Here's how the part is built. I have some questions about the finished solid (model axes, mm). A direction names the side the tool comes from. Round coordinates to 2 decimals unless told otherwise and drop trailing zeros. Loops run counter-clockwise (first coordinate to the right, second up) from the corner with the lowest first, then second, coordinate; pieces in that order, holes last. Notation, with made-up numbers: (56, 52) -> (72, 52) arc R30 cw to (72, 80) -> close; hole circle Ø5 at (69.5, 31.25). An arc over 180 degrees is marked (long way). Use one line per item in the form item = value. Start each with the question number.
Item 1: If we section it at C-C (z = 12.5): Write out the boundary of the cut face in (x, y), then the cut area to 3 significant figures.
Item 2: If we section it at D-D (z = 5): Write out the boundary of the cut face in (x, y), then the cut area to 3 significant figures.
Item 3: I'm going to push flat-ended pins straight in: pin 1 Ø1.5 at (y, z) = (-2.5, 12.5) entering from +X; pin 2 Ø8 at (y, z) = (-4.5, 9.5) entering from -X; pin 3 Ø3 at (x, z) = (2, 3.5) entering from +Y. Where does each tip first touch, or does it pass through?
Item 4: For faces 4 (the face through (-2.8, 0.1, 17.1)), 5 (the face through (-2.539, 1.947, 1.972)), which set-ups out of +Z, -Z, +X, -X, +Y, -Y let a thin tool reach every point of the face, with its end or its side?
Item 5: If I drill on L1, parallel to Y at x = 0, z = 13.75; L2, parallel to Y at x = 0, z = 8; L3, parallel to X at y = 1, z = 5.25, over which ranges is the centre line in solid material (lowest first)? Write a range as [from, to].
Item 6: Thinking about a two-plate mould opening in Y: for faces 1 (the face through (6.466, -2.681, 11.339)), 2 (the face through (1.5, -3, 0)), 3 (the face through (-3, 0, 7)), which applies, released by +Y, released by -Y, zero draft, split by the parting line, or undercut?
Item 7: If we section it at A-A (x = 0): Write out the boundary of the cut face in (y, z).
```python
from build123d import *

# Parameters (mm, degrees)
F0_R     = 7
F1_DEPTH = 23
F2_R     = 2.8
F3_DEPTH = 23.001
F4_R     = 3.2
F5_DEPTH = 4
F6_R     = 3
F7_DEPTH = 7


with BuildPart() as f1:
    # F0 (on Top) → F1 (new body)
    with BuildSketch(Plane.XY):
        Circle(F0_R)
    extrude(amount=F1_DEPTH)

    # F2 (on face) → F3 (cut, through all)
    with BuildSketch(Plane.XY.offset(23)):
        Circle(F2_R)
    extrude(amount=-F3_DEPTH, mode=Mode.SUBTRACT)

    # F4 (on face) → F5 (cut)
    with BuildSketch(Plane(origin=(0, 0, 0), x_dir=(1, 0, 0), z_dir=(0, 0, -1))):
        Circle(F4_R)
    extrude(amount=-F5_DEPTH, mode=Mode.SUBTRACT)

    # F6 (on face) → F7 (cut)
    with BuildSketch(Plane(origin=(0, 0, 4), x_dir=(1, 0, 0), z_dir=(0, 0, -1))):
        Circle(F6_R)
    extrude(amount=-F7_DEPTH, mode=Mode.SUBTRACT)


solid = f1.part
```
Values found:
q1.outline = circle Ø14 at (0, 0); hole circle Ø5.6 at (0, 0)
q1.area = 129 mm2
q2.outline = circle Ø14 at (0, 0); hole circle Ø6 at (0, 0)
q2.area = 126 mm2
q3.pin_1 = 6.78
q3.pin_2 = -6.98
q3.pin_3 = 6.98
q4.face_4 = +Z, -Z
q4.face_5 = -Z
q5.L1 = [-7, -2.8], [2.8, 7]
q5.L2 = [-7, -3], [3, 7]
q5.L3 = [-6.93, -2.83], [2.83, 6.93]
q6.face_1 = split by the parting line
q6.face_2 = zero draft
q6.face_3 = undercut
q7.outline = (-7, 0) -> (-3.2, 0) -> (-3.2, 4) -> (-3, 4) -> (-3, 11) -> (-2.8, 11) -> (-2.8, 23) -> (-7, 23) -> close; (2.8, 11) -> (3, 11) -> (3, 4) -> (3.2, 4) -> (3.2, 0) -> (7, 0) -> (7, 23) -> (2.8, 23) -> close
